The drawing under review shows one solid part. Ordinate dimensions are in mm from its lowest x, y, z. Give positions to 0.01 mm unless a question says otherwise; leave off trailing zeros. Write each loop counter-clockwise with the first axis right and the second up, starting at its lowest first coordinate (ties: lowest second). Pieces come first, ordered by that corner, then holes. Notation, with made-up numbers: M 9,33 L 58,33 A26 ccw 58,67 Z; hole C 3,84 d3. An arc over 180 degrees is marked long. Use one line per item in the form item = value. Start each with the question number.
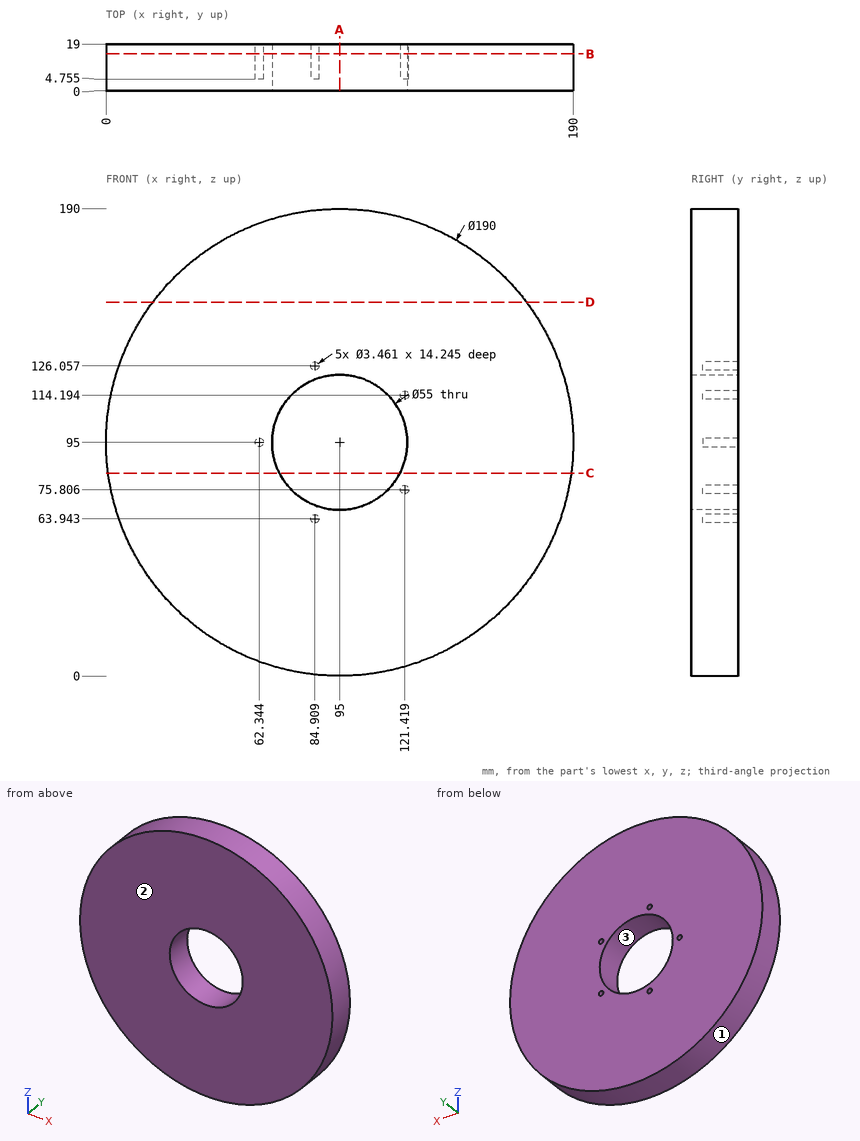
1. We need section B-B (y = 15). Give the number of separate pieces and of enclosed holes in the cut face, and give its area (3 significant figures).
2. To check wall thickness, follow L1, parallel to X at y = 12.75, z = 95 (1 decimal); L2, parallel to X at y = 16.5, z = 94.5 (1 decimal); L3, parallel to Z at x = 115.5, y = 16 (1 decimal). State the ranges of each line that lie inside material, in increasing order.
3. Clearance check with flat-ended pins moving along their axes: pin 1 Ø10 at (y, z) = (7.5, 134) entering from +X; pin 2 Ø4.5 at (x, z) = (62.34, 95) entering from +Y; pin 3 Ø1.5 at (y, z) = (10, 72.5) entering from -X; pin 4 Ø1.7 at (x, z) = (85.5, 64.5) entering from +Y (1 decimal). State where each tip first meets the part, or that it passes through.
4. Draft analysis for pull direction Z (two halves, no side actions). For the marked faces 1, 2 and 3, state which applies: pulls with the +Z half, pulls with the -Z half, needs draft (parallel to the pull), parting line crosses it, or undercut.
5. We need section D-D (z = 152). State the section outline as (x, y) points, and give its area (3 significant figures).
6. We need section A-A (x = 95). State the section outline as (y, z) points.
7. We need section C-C (z = 82.5). State the section outline as (x, y) points (1 decimal), and give its area (3 significant figures).
Answer block:
q1.separate_pieces = 1
q1.enclosed_holes = 6
q1.area = 25,900 mm^2
q2.L1 = 0 to 60.6, 64.1 to 67.5, 122.5 to 190
q2.L2 = 0 to 60.7, 64 to 67.5, 122.5 to 190
q2.L3 = 2.2 to 76.7, 113.3 to 187.8
q3.pin_1 = 183.71
q3.pin_2 = 19
q3.pin_3 = 2.52
q3.pin_4 = 4.8
q4.face_1 = parting line crosses it
q4.face_2 = needs draft
q4.face_3 = undercut
q5.outline = M 19,0 L 171,0 L 171,19 L 19,19 Z
q5.area = 2,890 mm^2
q6.outline = M 0,0 L 19,0 L 19,67.5 L 0,67.5 Z; M 0,122.5 L 19,122.5 L 19,190 L 0,190 Z
q7.outline = M 0.8,0 L 70.5,0 L 70.5,19 L 0.8,19 Z; M 119.5,0 L 189.2,0 L 189.2,19 L 119.5,19 Z
q7.area = 2,650 mm^2
